Verification items for the finished model (mm, model axes). A direction names the side the tool comes from. Round coordinates to 2 decimals unless told otherwise and drop trailing zeros. Loops run counter-clockwise (first coordinate to the right, second up) from the corner with the lowest first, then second, coordinate; pieces in that order, holes last. Notation, with made-up numbers: (79.25, 37) -> (122.25, 37) arc R27 ccw to (122.25, 64) -> close; hole circle Ø3 at (32.5, 43.5). An arc over 180 degrees is marked (long way). Use a Markdown table: item, result. Add a question column.
```python
from build123d import *

# Parameters (mm, degrees)
F1_DEPTH = 16
F2_W     = 3
F2_H     = 2
F3_DEPTH = 58
F4_W     = 10
F4_H     = 2
F6_F1_R  = 0.9999
F7_R     = 1
F8_R     = 2
F9_R     = 3


# Not quite as in the source:
# - a fillet or chamfer is up to 0.001 mm smaller than in the source, because OpenCascade refuses the exact size


with BuildPart() as f1:
    # F0 (on Right) → F1 (new body)
    with BuildSketch(Plane.YZ):
        Polygon((-61.7935170661, -87.8824494406), (-61.7935170661, -143.6097221679), (-81.7935170661, -120.8824494406), (-86.4557482916, -120.8824494406), (-64.4557482916, -145.8824494406), (-59.7935170661, -145.8824494406), (-59.7935170661, -89.8824494406), (-53.7935170661, -89.8824494406), (-53.7935170661, -117.8824494406), (-51.7935170661, -117.8824494406), (-51.7935170661, -87.8824494406), align=None)
    extrude(amount=F1_DEPTH)

    # F2 (on face) → F3 (join)
    with BuildSketch(Plane.XY.offset(-87.8824494406)):
        with Locations((1.5, -62.7935170661)):
            Rectangle(F2_W, F2_H)
        with Locations((14.5, -62.7935170661)):
            Rectangle(F2_W, F2_H)
    extrude(amount=-F3_DEPTH)

    # F5: sweep along a path in F5_path
    with BuildLine(Plane(origin=(16, -64.4557482916, -145.8824494406), x_dir=(0, 0.6606278949, -0.7507135169), z_dir=(0, 0.7507135169, 0.6606278949))) as f5_path:
        Line((0, 0), (-33.3016516107, 0))
    # F4 (on face) → F5 (sweep, cut)
    with BuildSketch(Plane.XY.offset(-120.8824494406)):
        with Locations((8, -85.4557482916)):
            Rectangle(F4_W, F4_H)
    sweep(path=f5_path.line, mode=Mode.SUBTRACT)

    # F6: fillet of radius 1 on 2 edges, made by hand

    # F6_f1 (radius 1 in the source; OpenCascade refuses exactly that, so slightly less here)
    f6_f1_edges = [f1.edges().sort_by_distance(p)[0] for p in [
        (1.5, -86.4557482916, -120.8824494406),
    ]]
    fillet(f6_f1_edges, radius=F6_F1_R)

    # F7
    f7_edges = [f1.edges().sort_by_distance(p)[0] for p in [
        (8, -81.793517, -120.882449),
    ]]
    fillet(f7_edges, radius=F7_R)

    # F8
    f8_edges = [f1.edges().sort_by_distance(p)[0] for p in [
        (14.5, -63.793517, -87.882449),
        (1.5, -63.793517, -87.882449),
    ]]
    fillet(f8_edges, radius=F8_R)

    # F9
    f9_edges = [f1.edges().sort_by_distance(p)[0] for p in [
        (14.5, -63.793517, -141.336995),
        (1.5, -63.793517, -141.336995),
    ]]
    fillet(f9_edges, radius=F9_R)


solid = f1.part
```
1) Access from +Z, -Z, +X, -X, +Y, -Y to the whole of each face (thin tool, end or side, straight path). Record for faces 4 (the face through (8, -57, -89.882)), 5 (the face through (8, -83, -120.882)), 6 (the face through (3, -74, -134)), 7 (the face through (3, -63, -118)).
2) Sectioned sample at A-A on z = -99.5. Enter the section's corners in (x, y), then the cut area to 3 significant figures.
3) Sectioned sample at B-B on x = 7.75. Enter the section's corners in (y, z), then the cut area to 3 significant figures.
4) Thickness scan on line 1 (Y direction, x = 11.5, z = -109.5); line 2 (Y direction, x = 2.75, z = -98); line 3 (Z direction, x = 5.25, y = -55). Record the ranges inside material, lowest first.
5) Release check for a two-part mould opening along X. For faces 1 (the face through (7.89, -73.7, -130.08)), 2 (the face through (0, -63.6, -118.9)), 3 (the face through (1, -63.794, -111)) record: released by +X, released by -X, zero draft, split by the parting line, or undercut.
6) Sectioned sample at C-C on y = -67. Enter the section's corners in (x, z), then the cut area to 3 significant figures.
7) Sectioned sample at D-D on z = -140. Enter the section's corners in (x, y).
8) Go/stop test with flat-tipped pins: pin 1 (1 mm diameter, centred on x = 4, z = -136.5, fed in from -Y); pin 2 (1.6 mm diameter, centred on x = 8.5, y = -83, fed in from +Z); pin 3 (4 mm diameter, centred on x = 7.5, y = -67.5, fed in from -Z). Record where each tip stops, or that it passes through.
Geometry results:
| question | item | result |
|---|---|---|
| 1 | face 4 | -Z, +X, -X |
| 1 | face 5 | +Z, +X, -X, -Y |
| 1 | face 6 | -Z, -Y |
| 1 | face 7 | +Z |
| 2 | outline | (0, -63.79) -> (3, -63.79) -> (3, -61.79) -> (13, -61.79) -> (13, -63.79) -> (16, -63.79) -> (16, -59.79) -> (0, -59.79) -> close; (0, -53.79) -> (16, -53.79) -> (16, -51.79) -> (0, -51.79) -> close |
| 2 | area | 76.0 mm^2 |
| 3 | outline | (-84.44, -120.9) -> (-62.46, -145.88) -> (-59.79, -145.88) -> (-59.79, -89.88) -> (-53.79, -89.88) -> (-53.79, -117.88) -> (-51.79, -117.88) -> (-51.79, -87.88) -> (-61.79, -87.88) -> (-61.79, -143.61) -> (-81.49, -121.22) arc R1 ccw to (-82.25, -120.88) -> (-84.24, -120.88) arc R1 ccw to start |
| 3 | area | 252 mm^2 |
| 4 | line 1 | -61.79 to -59.79, -53.79 to -51.79 |
| 4 | line 2 | -63.79 to -59.79, -53.79 to -51.79 |
| 4 | line 3 | -89.88 to -87.88 |
| 5 | face 1 | undercut |
| 5 | face 2 | released by -X |
| 5 | face 3 | zero draft |
| 6 | outline | (0, -142.99) -> (3, -142.99) -> (3, -140.72) -> (13, -140.72) -> (13, -142.99) -> (16, -142.99) -> (16, -136.38) -> (13, -136.38) -> (13, -137.69) -> (3, -137.69) -> (3, -136.38) -> (0, -136.38) -> close |
| 6 | area | 69.9 mm^2 |
| 7 | outline | (0, -69.63) -> (3, -69.63) -> (3, -67.63) -> (13, -67.63) -> (13, -69.63) -> (16, -69.63) -> (16, -59.79) -> (0, -59.79) -> close; hole (3, -64.97) -> (13, -64.97) -> (13, -61.79) -> (3, -61.79) -> close |
| 8 | pin 1 | y = -71.15 |
| 8 | pin 2 | z = -120.88 |
| 8 | pin 3 | z = -142.42 |
